from build123d import *

# Parameters (mm, degrees)
F1_DEPTH  = 45
F2_W      = 37
F2_H      = 11.55
F3_DEPTH  = 2
F4_R      = 3
F5_W      = 30.5
F5_H      = 10
F6_DEPTH  = 30.5
F7_R      = 14.25
F8_DEPTH  = 8.5
F10_W     = 20
F10_H     = 7.113087
F11_DEPTH = 25.4
F12_W     = 5.534876
F12_H     = 25.616745
F13_DEPTH = 2.5
F14_W     = 9.670809
F14_H     = 9.330716
F15_DEPTH = 25.4


with BuildPart() as f1:
    # F0 (on Right) → F1 (new body)
    with BuildSketch(Plane.YZ):
        Polygon((-35, 8), (-37.193318, 4), (-39.387777, 0), (-4.386635, 0), (-2.193318, 4), (0, 8), align=None)
    extrude(amount=F1_DEPTH)

    # F2 (on face) → F3 (cut)
    with BuildSketch(Plane.XY.offset(8)):
        with Locations((22.725, -26.922163)):
            Rectangle(F2_W, F2_H)
    extrude(amount=-F3_DEPTH, mode=Mode.SUBTRACT)

    # F4
    f4_edges = [f1.edges().sort_by_distance(p)[0] for p in [
        (4.225, -21.147163, 7),
        (4.225, -32.697163, 7),
        (41.225, -21.147163, 7),
        (41.225, -32.697163, 7),
    ]]
    fillet(f4_edges, radius=F4_R)

    # F5 (on face) → F6 (join)
    with BuildSketch(Plane.XY.offset(8)):
        with Locations((22.5, -16.147163)):
            Rectangle(F5_W, F5_H)
    extrude(amount=F6_DEPTH)

    # F7 (on face) → F8 (cut)
    with BuildSketch(Plane.XZ.offset(21.147163)):
        with Locations((22.506247, 23.256247)):
            Circle(F7_R)
    extrude(amount=-F8_DEPTH, mode=Mode.SUBTRACT)

    # F10 (on offset) → F11 (cut)
    with BuildSketch(Plane.XY.offset(12.319)):
        with Locations((22.506516, -21.107878)):
            Rectangle(F10_W, F10_H)
    extrude(amount=-F11_DEPTH, mode=Mode.SUBTRACT)

    # F12 (on face) → F13 (cut)
    with BuildSketch(Plane(origin=(0, 0, 0), x_dir=(1, 0, 0), z_dir=(0, 0, -1))):
        with Locations((22.506516, 4.771188)):
            Rectangle(F12_W, F12_H)
    extrude(amount=-F13_DEPTH, mode=Mode.SUBTRACT)

    # F14 (on offset) → F15 (cut)
    with BuildSketch(Plane.XY.offset(12.319)):
        with Locations((21.799793, -18.280461)):
            Rectangle(F14_W, F14_H)
    extrude(amount=-F15_DEPTH, mode=Mode.SUBTRACT)


solid = f1.part
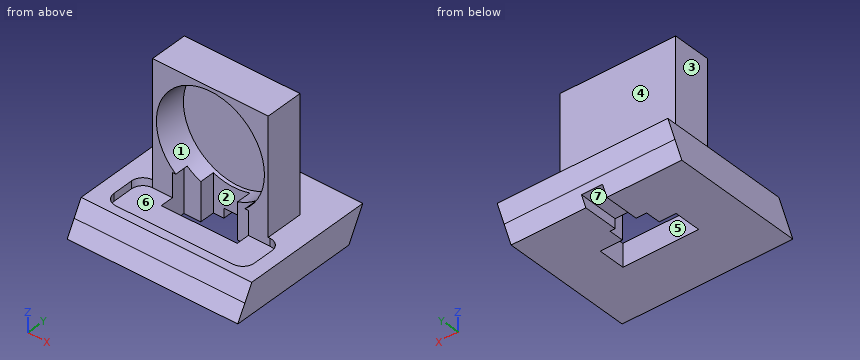
Model file for the job. Use its own axes, mm. Face numbers are marked on the shaded views. A direction names the side the tool comes from. Give positions to 0.01 mm unless a question says otherwise; leave off trailing zeros. Order: outer loops, then holes, each group sorted by start corner. A loop starts at its lowest first (then second) coordinate and runs counter-clockwise, first axis right, second up. Notation, with made-up numbers: (4.25, 76) - (16.25, 76) arc R27 ccw to (16.25, 101) - close; hole circle Ø1 at (16.5, 88). An arc over 180 degrees is marked (long way). Return JSON: item names as keys, results as strings.
1) Cut at A-A, the plane y = -15.5. Give the cut face in (x, z), plus the area to 3 significant figures.
Geometry says:
{"outline": "(0, 0) - (16.96, 0) - (16.96, 10.13) arc R14.25 cw (long way) to (26.64, 9.62) - (26.64, 0) - (45, 0) - (45, 8) - (37.75, 8) - (37.75, 38.5) - (7.25, 38.5) - (7.25, 8) - (0, 8) - close", "area": "562 mm²"}
2) 3-axis set-ups, long thin cutter, end or side, ignore diameter. For the marked faces 1, 2 and 3: which of +Z, -Z, +X, -X, +Y, -Y reach the whole face in a straight line?
Geometry says:
{"face 1": "-Y", "face 2": "-Z", "face 3": "+Z, -X, +Y, -Y"}
3) Cut at C-C, the plane z = 20.5. Give the cut face in (x, y).
Geometry says:
{"outline": "(7.25, -21.15) - (8.53, -21.15) - (8.53, -12.65) - (36.49, -12.65) - (36.49, -21.15) - (37.75, -21.15) - (37.75, -11.15) - (7.25, -11.15) - close"}
4) Pull direction Y, two halves, no side cores. Call the marked faces 4, 5, 6 and 7: pulls with the +Y half, pulls with the -Y half, needs draft (parallel to the pull), parting line crosses it, or undercut.
Geometry says:
{"face 4": "pulls with the +Y half", "face 5": "undercut", "face 6": "undercut", "face 7": "needs draft"}
5) Probe line 1 (X direction, y = -18.5, z = 21.5); line 2 (Y direction, x = 18, z = 30.5); line 3 (Z direction, x = 11, y = -27). List the from-to ranges inside material, lowest first. Write a range as from..to.
Geometry says:
{"line 1": "7.25..8.36, 36.65..37.75", "line 2": "-12.65..-11.15", "line 3": "0..6"}
6) Cut at D-D, the plane y = -27. Give the cut face in (x, z) (3 decimals), plus the area to 3 significant figures.
Geometry says:
{"outline": "(0, 0) - (45, 0) - (45, 8) - (41.225, 8) - (41.225, 6) - (4.225, 6) - (4.225, 8) - (0, 8) - close", "area": "286 mm²"}
7) Cut at B-B, the plane x = 34.5. Give the cut face in (y, z), plus the area to 3 significant figures.
Geometry says:
{"outline": "(-39.39, 0) - (-4.39, 0) - (-2.19, 4) - (0, 8) - (-11.15, 8) - (-11.15, 38.5) - (-21.15, 38.5) - (-21.15, 30.95) - (-12.65, 30.95) - (-12.65, 15.56) - (-21.15, 15.56) - (-21.15, 6) - (-32.7, 6) - (-32.7, 8) - (-35, 8) - (-37.19, 4) - close", "area": "431 mm²"}
8) Flat gauge pins, fed straight in: P1, Ø9.5, axis at x = 17.5, z = 30.5, coming from the -Y side; P2, Ø10, axis at y = -16.5, z = 29, coming from the -X side; P3, Ø4, axis at x = 38.5, z = 14.5, coming from the -Y side; P4, Ø1, axis at x = 40, z = 12.5, coming from the +Y side. Where does each tip first touch, or does it go through?
Geometry says:
{"P1": "y = -12.65", "P2": "x = 7.25", "P3": "y = -21.15", "P4": "through"}
